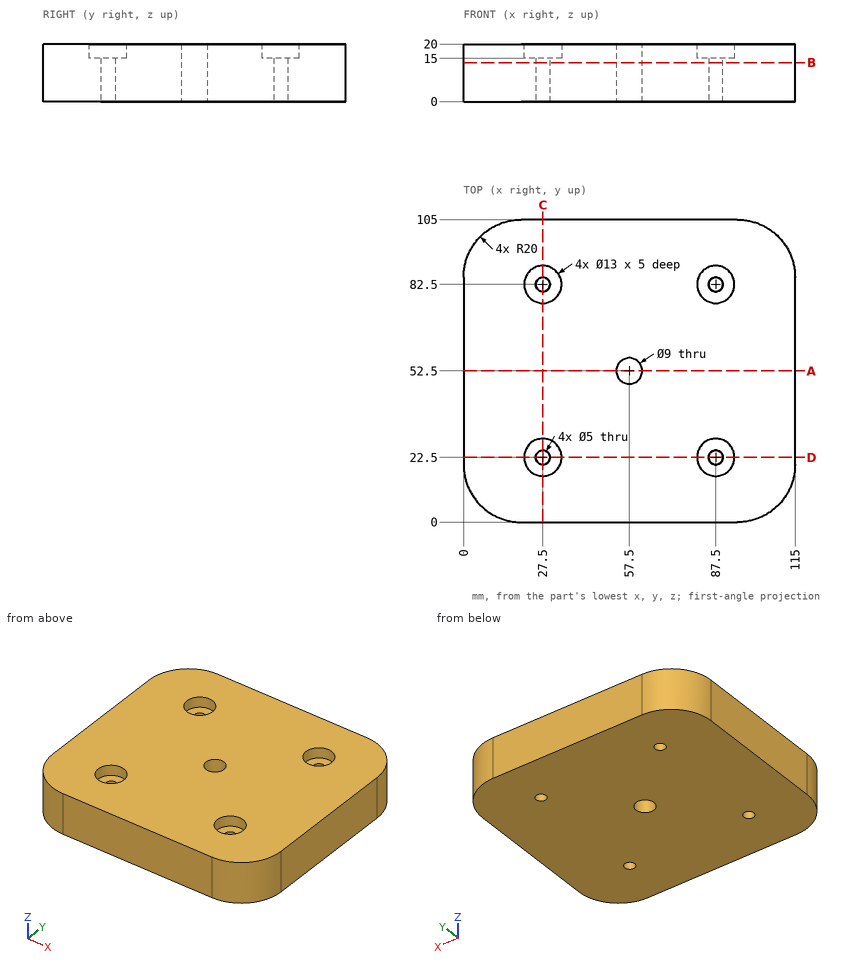
Here's the drawing with two shaded views (mm, measured from the low corner). I have some questions. Round coordinates to 2 decimals unless told otherwise and drop trailing zeros. Order: outer loops, then holes, each group sorted by start corner. A loop starts at its lowest first (then second) coordinate and runs counter-clockwise, first axis right, second up. Notation, with made-up numbers: (16.5, 71.25) -> (46.5, 71.25) arc R31 cw to (46.5, 96.25) -> close; hole circle Ø4 at (-23, 29.5). An arc over 180 degrees is marked (long way). Use a Markdown table: item, result. Add a question column.
(1) Suppose I cut it at C-C, the plane x = 27.5. Please give me the cut outline in (y, z), and give its area (3 significant figures).
(2) I need wall thicknesses on line 1 along X through (y, z) = (22.5, 11.25); line 2 along Y through (x, z) = (27.5, 16.8); line 3 along Y through (x, z) = (27.5, 7.5). Which ranges of each line are inside material? Lowest first, please.
(3) Suppose I cut it at A-A, the plane y = 52.5. Please give me the cut outline in (x, z).
(4) For pin 1 Ø6.5 at (x, y) = (87.5, 22.5) entering from +Z, with a flat end and sliding along its axis, tell me the tip position at first contact or that it passes through.
(5) Suppose I cut it at D-D, the plane y = 22.5. Please give me the cut outline in (x, z).
(6) Suppose I cut it at B-B, the plane z = 13.5. Please give me the cut outline in (x, y).
Verdict:
| question | item | result |
|---|---|---|
| 1 | outline | (0, 0) -> (20, 0) -> (20, 15) -> (16, 15) -> (16, 20) -> (0, 20) -> close; (25, 0) -> (80, 0) -> (80, 15) -> (76, 15) -> (76, 20) -> (29, 20) -> (29, 15) -> (25, 15) -> close; (85, 0) -> (105, 0) -> (105, 20) -> (89, 20) -> (89, 15) -> (85, 15) -> close |
| 1 | area | 1,820 mm2 |
| 2 | line 1 | 0 to 25, 30 to 85, 90 to 115 |
| 2 | line 2 | 0 to 16, 29 to 76, 89 to 105 |
| 2 | line 3 | 0 to 20, 25 to 80, 85 to 105 |
| 3 | outline | (0, 0) -> (53, 0) -> (53, 20) -> (0, 20) -> close; (62, 0) -> (115, 0) -> (115, 20) -> (62, 20) -> close |
| 4 | pin 1 | z = 15 |
| 5 | outline | (0, 0) -> (25, 0) -> (25, 15) -> (21, 15) -> (21, 20) -> (0, 20) -> close; (30, 0) -> (85, 0) -> (85, 15) -> (81, 15) -> (81, 20) -> (34, 20) -> (34, 15) -> (30, 15) -> close; (90, 0) -> (115, 0) -> (115, 20) -> (94, 20) -> (94, 15) -> (90, 15) -> close |
| 6 | outline | (0, 20) arc R20 ccw to (20, 0) -> (95, 0) arc R20 ccw to (115, 20) -> (115, 85) arc R20 ccw to (95, 105) -> (20, 105) arc R20 ccw to (0, 85) -> close; hole circle Ø5 at (27.5, 22.5); hole circle Ø5 at (27.5, 82.5); hole circle Ø9 at (57.5, 52.5); hole circle Ø5 at (87.5, 22.5); hole circle Ø5 at (87.5, 82.5) |
